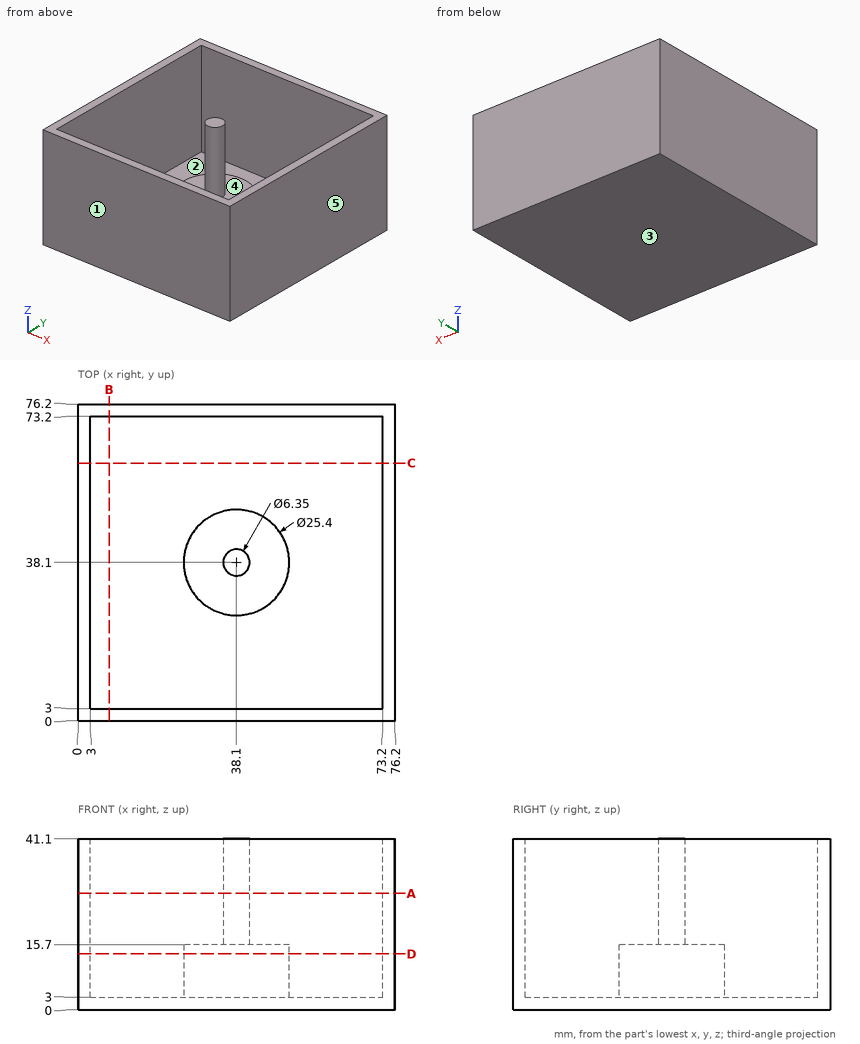
Design review of the part shown in the three views and the two pictorial views. Dimensions are in mm from the part's minimum x, y and z. A direction names the side the tool comes from. Round coordinates to 2 decimals unless told otherwise and drop trailing zeros. Write each loop counter-clockwise with the first axis right and the second up, starting at its lowest first coordinate (ties: lowest second). Pieces come first, ordered by that corner, then holes. Notation, with made-up numbers: M -24.5,60 L -0.5,60 A20 ccw -0.5,94 Z; hole C 50.5,64 d4. An arc over 180 degrees is marked long. One line per item, written item: value. Start each with the question number.
1. Take a section at A-A on z = 28. State the section outline as (x, y) points (3 decimals), then the cut area to 3 significant figures.
2. Take a section at D-D on z = 13.5. State the section outline as (x, y) points.
3. Draft analysis for pull direction Y (two halves, no side actions). For the marked faces 1, 2 and 3, state which applies: pulls with the +Y half, pulls with the -Y half, needs draft (parallel to the pull), parting line crosses it, or undercut.
4. Clearance check with flat-ended pins moving along their axes: P1, Ø20.5, axis at x = 33, y = 35, coming from the +Z side; P2, Ø6, axis at x = 30, y = 64.5, coming from the +Z side. State where each tip first meets the part, or that it passes through.
5. Take a section at B-B on x = 7.5. State the section outline as (y, z) points.
6. For the marked faces 4 and 5, list the 3-axis set-ups (+Z, -Z, +X, -X, +Y, -Y) from which the entire face can be reached by the end or side of a thin tool; tool diameter is ignored.
7. To check wall thickness, follow probe 1 along Y at (x, z) = (18.5, 3.5); probe 2 along Z at (x, y) = (37, 33). State the ranges of each line that lie inside material, in increasing order. Write a range as from..to.
Computed:
1. outline: M 0,0 L 76.2,0 L 76.2,76.2 L 0,76.2 Z; C 38.1,38.1 d6.35; hole M 3,3 L 73.2,3 L 73.2,73.2 L 3,73.2 Z
1. area: 910 mm²
2. outline: M 0,0 L 76.2,0 L 76.2,76.2 L 0,76.2 Z; C 38.1,38.1 d25.4; hole M 3,3 L 73.2,3 L 73.2,73.2 L 3,73.2 Z
3. face 1: pulls with the -Y half
3. face 2: undercut
3. face 3: needs draft
4. P1: stops at z = 41.1
4. P2: stops at z = 3
5. outline: M 0,0 L 76.2,0 L 76.2,41.1 L 73.2,41.1 L 73.2,3 L 3,3 L 3,41.1 L 0,41.1 Z
6. face 4: +Z
6. face 5: +Z, -Z, +X, +Y, -Y
7. probe 1: y = 0..3, 73.2..76.2
7. probe 2: z = 0..15.7
